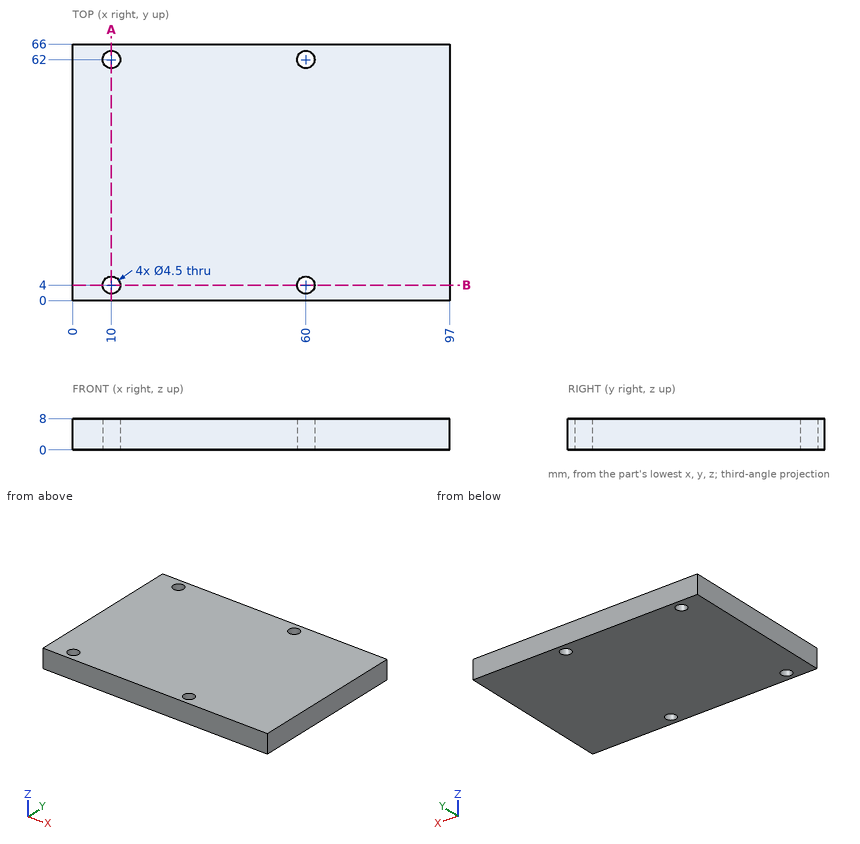
Study the drawing (mm; zero at the part's minimum x, y, z) and answer. Coordinates: 2 decimals unless noted, no trailing zeros. Write each loop counter-clockwise with the first axis right and the second up, starting at its lowest first coordinate (ties: lowest second). Pieces come first, ordered by that corner, then holes. Notation, with made-up numbers: (68, -24.5) - (109, -24.5) arc R6 ccw to (109, -15.5) - close; hole circle Ø3 at (-15.5, 77.25). An arc over 180 degrees is marked (long way). Put each result on its own line as item: value.
1. The part is cut by section A-A on x = 10. Give the vertices of the cut face in (y, z), plus the area to 3 significant figures.
Answer sheet:
outline: (0, 0) - (1.75, 0) - (1.75, 8) - (0, 8) - close; (6.25, 0) - (59.75, 0) - (59.75, 8) - (6.25, 8) - close; (64.25, 0) - (66, 0) - (66, 8) - (64.25, 8) - close
area: 456 mm^2
2. Find the intervals of material crossed by line 1 along Y through (x, z) = (60, 2.5); line 2 along X through (y, z) = (62, 4.75), in increasing order. Write a range as from..to.
Answer sheet:
line 1: y = 0..1.75, 6.25..59.75, 64.25..66
line 2: x = 0..7.75, 12.25..57.75, 62.25..97
3. The part is cut by section B-B on y = 4. Give the vertices of the cut face in (x, z), plus the area to 3 significant figures.
Answer sheet:
outline: (0, 0) - (7.75, 0) - (7.75, 8) - (0, 8) - close; (12.25, 0) - (57.75, 0) - (57.75, 8) - (12.25, 8) - close; (62.25, 0) - (97, 0) - (97, 8) - (62.25, 8) - close
area: 704 mm^2
